Here's how the part is built. I have some questions about the finished solid (model axes, mm). A direction names the side the tool comes from. Coordinates: 2 decimals unless noted, no trailing zeros. Loops run counter-clockwise (first coordinate to the right, second up) from the corner with the lowest first, then second, coordinate; pieces in that order, holes last.
```python
from build123d import *

# Parameters (mm, degrees)
F1_DEPTH = 38
F2_R     = 19.5
F3_DEPTH = 26
F5_DEPTH = 93
F7_DEPTH = 34.501


with BuildPart() as f1:
    # F0 (on Top) → F1 (new body)
    with BuildSketch(Plane.XY):
        with BuildLine():
            Line((8.170067, 21.5), (-8.170067, 21.5))
            ThreePointArc((-8.170067, 21.5), (-23, 0), (-8.170067, -21.5))
            Line((-8.170067, -21.5), (8.170067, -21.5))
            ThreePointArc((8.170067, -21.5), (23, 0), (8.170067, 21.5))
        make_face()
    extrude(amount=F1_DEPTH)

    # F2 (on face) → F3 (cut)
    with BuildSketch(Plane.XY.offset(38)):
        Circle(F2_R)
    extrude(amount=-F3_DEPTH, mode=Mode.SUBTRACT)

    # F4 (on face) → F5 (join)
    with BuildSketch(Plane(origin=(0, 0, 0), x_dir=(1, 0, 0), z_dir=(0, 0, -1))):
        with BuildLine():
            Line((-11.5, 15.748016), (-11.5, -15.748016))
            ThreePointArc((-11.5, -15.748016), (0, -19.5), (11.5, -15.748016))
            Line((11.5, -15.748016), (11.5, 15.748016))
            ThreePointArc((11.5, 15.748016), (0, 19.5), (-11.5, 15.748016))
        make_face()
    extrude(amount=F5_DEPTH)

    # F6 (on face) → F7 (cut, through all)
    with BuildSketch(Plane(origin=(-11.5, 0, 0), x_dir=(0, -1, 0), z_dir=(-1, 0, 0))):
        with BuildLine():
            Line((38.116675, -101.656117), (19.472977, -82.23941))
            ThreePointArc((19.472977, -82.23941), (17.755152, -84.620348), (15.748016, -86.763055))
            Line((15.748016, -86.763055), (15.748016, -93))
            Line((15.748016, -93), (0, -93))
            Line((0, -93), (-15.748016, -93))
            Line((-15.748016, -93), (-15.748016, -86.763055))
            ThreePointArc((-15.748016, -86.763055), (-17.850565, -84.503701), (-19.63169, -81.983187))
            Line((-19.63169, -81.983187), (-36.674619, -101.656117))
            Line((-36.674619, -101.656117), (38.116675, -101.656117))
        make_face()
        with BuildLine():
            Line((15.748016, -93), (15.748016, -86.763055))
            ThreePointArc((15.748016, -86.763055), (8.469054, -91.383992), (0, -93))
            Line((0, -93), (15.748016, -93))
        make_face()
        with BuildLine():
            Line((-15.748016, -93), (0, -93))
            ThreePointArc((0, -93), (-8.469054, -91.383992), (-15.748016, -86.763055))
            Line((-15.748016, -86.763055), (-15.748016, -93))
        make_face()
    extrude(amount=-F7_DEPTH, mode=Mode.SUBTRACT)


solid = f1.part
```
1. I want a section at D-D (x = -14.5). Please give me the cut outline in (y, z), then the cut area to 3 significant figures.
2. I need wall thicknesses on line 1 along Z through (x, y) = (-16, 16); line 2 along Y through (x, z) = (-3.5, 20); line 3 along Y through (x, z) = (0, 22.75). Which ranges of each line are inside material? Lowest first, please.
3. I want a section at B-B (y = -7). Please give me the cut outline in (x, z), then the cut area to 3 significant figures.
4. I want a section at A-A (z = 24.5). Please give me the cut outline in (x, y), then the cut area to 3 significant figures.
5. We'd pull the mould along X, two halves only. Please class faces 1 (the flat face through (0, 0, 12)), 2 (the cylindrical face through (-0.161, 17.319, -85.135)), 3 (the cylindrical face through (-23, 0, 19)): +X half, -X half, draft (parallel to the pull), parting line (faces both ways), or undercut.
6. For pin 1 (15.5 mm diameter, centred on y = 7.5, z = -57.5, fed in from -X); pin 2 (8 mm diameter, centred on y = -17, z = -41, fed in from +X); pin 3 (12 mm diameter, centred on x = -9, z = -48.5, fed in from -Y), each with a flat end and sliding along its axis, tell me the tip position at first contact or that it passes through.
7. On a 3-axis mill with a long thin cutter (end or side, diameter ignored), from which of +Z, -Z, +X, -X, +Y, -Y can I reach the whole of each face in a straight line? I mean faces 4 (the cylindrical face through (-2.539, 19.334, 25.182)), 5 (the flat face through (-11.5, 0, -46)), 6 (the flat face through (11.5, 0, -46)), 7 (the cylindrical face through (0.2, -19.5, -42.8)). Say none if no direction works.
8. I want a section at C-C (z = -84). Please give me the cut outline in (x, y).
Response values:
1. outline: (-17.85, 0) - (17.85, 0) - (17.85, 38) - (13.04, 38) - (13.04, 12) - (-13.04, 12) - (-13.04, 38) - (-17.85, 38) - close
1. area: 679 mm2
2. line 1: z = 0 to 38
2. line 2: y = -21.5 to -19.18, 19.18 to 21.5
2. line 3: y = -21.5 to -19.5, 19.5 to 21.5
3. outline: (-21.91, 0) - (-11.5, 0) - (-11.5, -91.91) - (11.5, -91.91) - (11.5, 0) - (21.91, 0) - (21.91, 38) - (18.2, 38) - (18.2, 12) - (-18.2, 12) - (-18.2, 38) - (-21.91, 38) - close
3. area: 2,830 mm2
4. outline: (-8.17, -21.5) - (8.17, -21.5) arc R23 ccw to (8.17, 21.5) - (-8.17, 21.5) arc R23 ccw to start; hole circle Ø39 at (0, 0)
4. area: 434 mm2
5. face 1: undercut
5. face 2: draft
5. face 3: -X half
6. pin 1: stops at x = -11.5
6. pin 2: stops at x = 11.5
6. pin 3: stops at y = -19.27
7. face 4: +Z
7. face 5: -Z, -X, +Y, -Y
7. face 6: -Z, +X, +Y, -Y
7. face 7: -Z, -Y
8. outline: (-11.5, -15.75) arc R19.5 ccw to (-6.87, -18.25) - (6.87, -18.25) arc R19.5 ccw to (11.5, -15.75) - (11.5, 15.75) arc R19.5 ccw to (6.87, 18.25) - (-6.87, 18.25) arc R19.5 ccw to (-11.5, 15.75) - close
